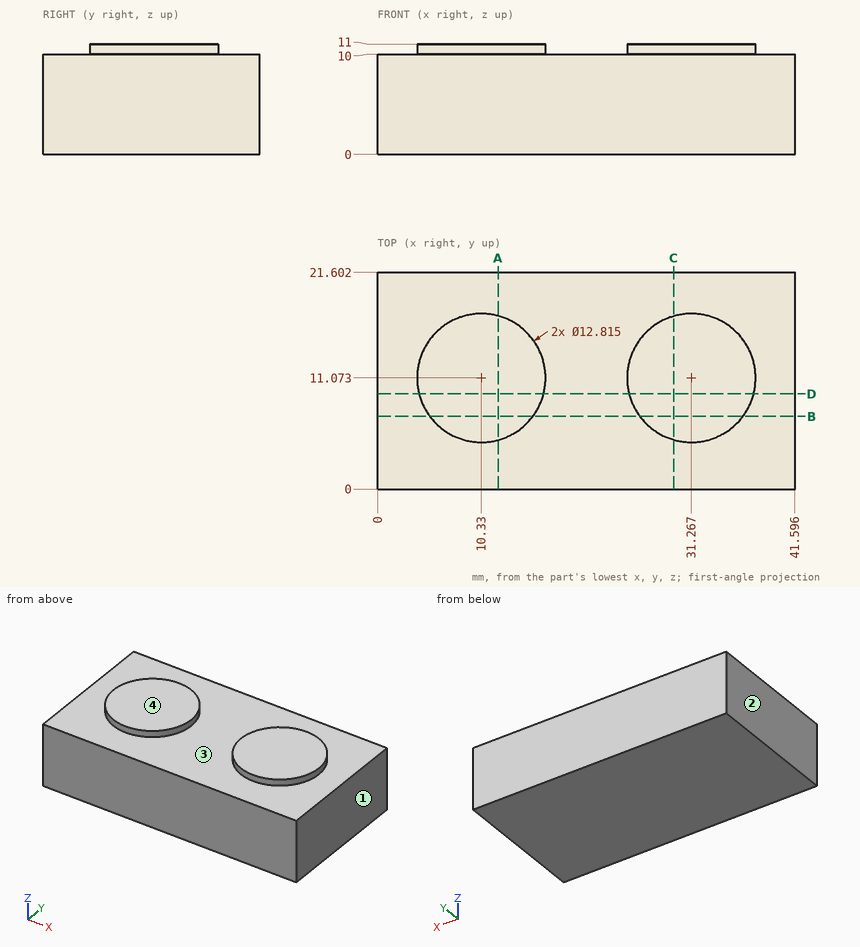
Print and shaded views of the part. All mm, measured from the part's lowest x, y and z. Give positions to 0.01 mm unless a question says otherwise; leave off trailing zeros. Order: outer loops, then holes, each group sorted by start corner. A loop starts at its lowest first (then second) coordinate and runs counter-clockwise, first axis right, second up. Notation, with made-up numbers: (29, 87) - (47, 87) arc R35 ccw to (47, 120) - close; hole circle Ø6 at (-23.5, 1.5). An arc over 180 degrees is marked (long way). One line per item, written item: value.
Item 1: Slice it at D-D (y = 9.5). List the corners of the cut face in (x, z) (1 decimal), then the cut area to 3 significant figures.
Response values:
outline: (0, 0) - (41.6, 0) - (41.6, 10) - (37.5, 10) - (37.5, 11) - (25.1, 11) - (25.1, 10) - (16.5, 10) - (16.5, 11) - (4.1, 11) - (4.1, 10) - (0, 10) - close
area: 441 mm2
Item 2: Wall check: line 1 (Z direction, x = 18.5, y = 15.5); line 2 (X direction, y = 15.5, z = 10.25) (1 decimal). Give the ranges that are in metal, low to high.
Response values:
line 1: 0 to 10
line 2: 5.7 to 15, 26.6 to 35.9
Item 3: Slice it at B-B (y = 7.25). List the corners of the cut face in (x, z) (1 decimal).
Response values:
outline: (0, 0) - (41.6, 0) - (41.6, 10) - (36.4, 10) - (36.4, 11) - (26.1, 11) - (26.1, 10) - (15.5, 10) - (15.5, 11) - (5.2, 11) - (5.2, 10) - (0, 10) - close
Item 4: Two-plate mould, pull along X, no slides. Class the marked faces 1, 2, 3 and 4: released by +X, released by -X, zero draft, split by the parting line, or undercut.
Response values:
face 1: released by +X
face 2: released by -X
face 3: undercut
face 4: zero draft
Item 5: Slice it at C-C (x = 29.5). List the corners of the cut face in (y, z).
Response values:
outline: (0, 0) - (21.6, 0) - (21.6, 10) - (17.23, 10) - (17.23, 11) - (4.91, 11) - (4.91, 10) - (0, 10) - close
Item 6: Slice it at A-A (x = 12). List the corners of the cut face in (y, z), then the cut area to 3 significant figures.
Response values:
outline: (0, 0) - (21.6, 0) - (21.6, 10) - (17.26, 10) - (17.26, 11) - (4.89, 11) - (4.89, 10) - (0, 10) - close
area: 228 mm2
